```python
from build123d import *

# Parameters (mm, degrees)
BASPROSKE_W             = 10
BASPROSKE_H             = 19
TOOTHCUT_DEPTH          = 29.670542374
TEETHCUTS_COUNT         = 17
TEETHCUTS_ANGLE         = 338.823529412
BORSKE_R                = 2.5
BORE_DEPTH              = 50.0019304
SKETCH1_W               = 10
SKETCH1_H               = 40
CUT_EXTRUDE1_DEPTH      = 20
CUT_EXTRUDE1_DEPTH_BACK = 20
BOSS_EXTRUDE1_DEPTH     = 5
SKETCH5_R               = 1.5
CUT_EXTRUDE5_DEPTH      = 68.251600881
FILLET2_R               = 4.5
SKETCH7_R               = 6
CUT_EXTRUDE7_DEPTH      = 3
CUT_EXTRUDE8_DEPTH      = 2
SKETCH8_R               = 1.5
CUT_EXTRUDE9_DEPTH      = 64.982759166
FILLET3_R               = 4.5


with BuildPart() as part:
    # BasProSke → Base-Revolve (revolve)
    with BuildSketch(Plane(origin=(0, 0, 0), x_dir=(1, 0, 0), z_dir=(0, 1, 0)), mode=Mode.PRIVATE) as base_revolve_sk:
        with Locations((5, 9.5)):
            Rectangle(BASPROSKE_W, BASPROSKE_H)
    revolve(base_revolve_sk.sketch.rotate(Axis((-10, 0, 0), (1, 0, 0)), 180), axis=Axis((-10, 0, 0), (1, 0, 0)))

    # TooCutSke → ToothCut (cut, through all)
    with BuildSketch(Plane(origin=(0, 0, 0), x_dir=(0, 0, -1), z_dir=(1, 0, 0))):
        with BuildLine():
            ThreePointArc((1.020352389, 14.463052306), (0, 14.499), (-1.020352389, 14.463052306))
            ThreePointArc((-1.020352389, 14.463052306), (-1.632621885, 16.804485203), (-3.026143023, 18.783192049))
            ThreePointArc((-3.026143023, 18.783192049), (0, 19.0254), (3.026143023, 18.783192049))
            ThreePointArc((3.026143023, 18.783192049), (1.632621885, 16.804485203), (1.020352389, 14.463052306))
        make_face()
    toothcut = extrude(amount=TOOTHCUT_DEPTH, mode=Mode.SUBTRACT)

    # TeethCuts: ToothCut ×17 about axis
    teethcuts_axis = Axis((-10, 0, 0), (1, 0, 0))
    for i in range(1, TEETHCUTS_COUNT):
        add(toothcut.rotate(teethcuts_axis, i * TEETHCUTS_ANGLE / (TEETHCUTS_COUNT - 1)), mode=Mode.SUBTRACT)

    # BorSke → Bore (cut, symmetric)
    with BuildSketch(Plane(origin=(0, 0, 0), x_dir=(0, 0, -1), z_dir=(1, 0, 0))):
        with Locations(Location((0, 0, 0), (0, 0, 180))):
            Circle(BORSKE_R)
    extrude(amount=BORE_DEPTH, both=True, mode=Mode.SUBTRACT)

    # Sketch1 → Cut-Extrude1 (cut, two sides)
    with BuildSketch(Plane.XY) as cut_extrude1_sk:
        Rectangle(SKETCH1_W, SKETCH1_H)
    extrude(amount=CUT_EXTRUDE1_DEPTH, mode=Mode.SUBTRACT)
    extrude(cut_extrude1_sk.sketch, amount=-CUT_EXTRUDE1_DEPTH_BACK, mode=Mode.SUBTRACT)

    # Sketch4 → Boss-Extrude1 (add)
    with BuildSketch(Plane(origin=(10, 0, 0), x_dir=(0, 0, -1), z_dir=(1, 0, 0))):
        with BuildLine():
            Line((5, 0), (5, 47.113248654))
            Line((5, 47.113248654), (14.820508076, 52.783121635))
            Line((14.820508076, 52.783121635), (14.820508076, 64.330127019))
            Line((14.820508076, 64.330127019), (-5, 52.886751346))
            Line((-5, 52.886751346), (-5, 0))
            Line((-5, 0), (-2.5, 0))
            ThreePointArc((-2.5, 0), (0, 2.5), (2.5, 0))
            Line((2.5, 0), (5, 0))
        make_face()
    extrude(amount=-BOSS_EXTRUDE1_DEPTH)

    # Sketch5 → Cut-Extrude5 (cut, through all)
    with BuildSketch(Plane.ZY.offset(-5)):
        with Locations(Location((-11.320508076, 57.330127019, 0), (0, 0, 270))):
            Circle(SKETCH5_R)
    extrude(amount=-CUT_EXTRUDE5_DEPTH, mode=Mode.SUBTRACT)

    # Fillet2
    fillet2_edges = [part.edges().sort_by_distance(p)[0] for p in [
        (7.5, 64.330127019, -14.820508076),
        (7.5, 52.783121635, -14.820508076),
    ]]
    fillet(fillet2_edges, radius=FILLET2_R)

    # Sketch7 → Cut-Extrude7 (cut)
    with BuildSketch(Plane(origin=(10, 0, 0), x_dir=(0, 0, -1), z_dir=(1, 0, 0))):
        with Locations((11.320508076, 57.330127019)):
            Circle(SKETCH7_R)
    extrude(amount=-CUT_EXTRUDE7_DEPTH, mode=Mode.SUBTRACT)

    # Sketch2 → Cut-Extrude8 (cut)
    with BuildSketch(Plane.ZY.offset(-5)):
        with BuildLine():
            Line((0, -12.5), (0, -4))
            ThreePointArc((0, -4), (-2.624080254, -3.018973803), (-3.961014771, -0.557101411))
            Line((-3.961014771, -0.557101411), (-2, -14.5))
            ThreePointArc((-2, -14.5), (-1.414213562, -13.085786438), (0, -12.5))
        make_face()
        with BuildLine():
            ThreePointArc((2, -14.5), (1.414213562, -13.085786438), (0, -12.5))
            Line((0, -12.5), (0, -16.5))
            ThreePointArc((0, -16.5), (1.414213562, -15.914213562), (2, -14.5))
        make_face()
        with BuildLine():
            Line((0, -16.5), (0, -12.5))
            ThreePointArc((0, -12.5), (-1.414213562, -13.085786438), (-2, -14.5))
            ThreePointArc((-2, -14.5), (-1.414213562, -15.914213562), (0, -16.5))
        make_face()
        with BuildLine():
            ThreePointArc((3.850641774, -1.082847141), (2.415430752, -3.188368593), (0, -4))
            Line((0, -4), (0, -12.5))
            ThreePointArc((0, -12.5), (1.414213562, -13.085786438), (2, -14.5))
            Line((2, -14.5), (3.850641774, -1.082847141))
        make_face()
        with BuildLine():
            ThreePointArc((-3.961014771, -0.557101411), (-2.624080254, -3.018973803), (0, -4))
            ThreePointArc((0, -4), (2.415430752, -3.188368593), (3.850641774, -1.082847141))
            Line((3.850641774, -1.082847141), (4, 0))
            ThreePointArc((4, 0), (-0.279231906, 3.99024179), (-3.961014771, -0.557101411))
        make_face()
        with BuildLine():
            ThreePointArc((2.5, 0), (1.767766953, -1.767766953), (0, -2.5))
            ThreePointArc((0, -2.5), (-1.767766953, 1.767766953), (2.5, 0))
        make_face(mode=Mode.SUBTRACT)
    extrude(amount=-CUT_EXTRUDE8_DEPTH, mode=Mode.SUBTRACT)

    # Sketch8 → Cut-Extrude9 (cut, through all)
    with BuildSketch(Plane.ZY.offset(-7)):
        with Locations(Location((0, -8.45, 0), (0, 0, 270))):
            Circle(SKETCH8_R)
        with Locations(Location((0, -12.45, 0), (0, 0, 270))):
            Circle(SKETCH8_R)
    extrude(amount=-CUT_EXTRUDE9_DEPTH, mode=Mode.SUBTRACT)

    # Fillet3
    fillet3_edges = [part.edges().sort_by_distance(p)[0] for p in [
        (8.5, 51.449252752, -12.5101794),
    ]]
    fillet(fillet3_edges, radius=FILLET3_R)


solid = part.part
```
Geometry check sheet. Reference: the model listing, model coordinates, mm. A direction names the side the tool comes from. Round coordinates to 2 decimals unless told otherwise and drop trailing zeros. Order: outer loops, then holes, each group sorted by start corner. A loop starts at its lowest first (then second) coordinate and runs counter-clockwise, first axis right, second up. Notation, with made-up numbers: (70, -1.5) - (106, -1.5) arc R11 ccw to (106, 7.5) - close; hole circle Ø7 at (25.25, 84). An arc over 180 degrees is marked (long way). Use a Markdown table: item, result. Add a question column.
(1) Sectioned sample at A-A, the plane y = 40. Enter the section's corners in (x, z), and give its area (3 significant figures).
(2) Tool access check on faces 4 (the cylindrical face through (7.46, 10.72, 9.76)), 5 (the cylindrical face through (7.465, -16.178, -4.664)), 6 (the flat face through (7, -6, 0)), 7 (the cylindrical face through (7.465, 1.352, 14.436)), 8 (the cylindrical face through (5.986, 53.16, -14.234)). Record the directions out of +Z, -Z, +X, -X, +Y, -Y that give a thin tool (end or side, any length) a straight path to the whole face; none if there is none.
(3) Release check for a two-part mould opening along Y. For faces 1 (the cylindrical face through (7.465, -15.098, 7.452)), 2 (the cylindrical face through (7.46, 11.3, 12.48)), 3 (the flat face through (8, 34, 5)) record: pulls with the +Y half, pulls with the -Y half, needs draft (parallel to the pull), parting line crosses it, or undercut.
(4) Sectioned sample at B-B, the plane x = 6. Count the separate pieces of the cut face and the enclosed holes in it, and give its area (3 significant figures).
(5) Material ranges on line 1 along Z through (x, y) = (7.95, -12.45); line 2 along Z through (x, y) = (9.3, -8.45); line 3 along Z through (x, y) = (5.6, -11.5), recorded low to high. Write a range as [from, to].
(6) Depth check by flat-ended pin: pin 1 (3 mm diameter, centred on y = 53.5, z = -11, fed in from +X); pin 2 (6.5 mm diameter, centred on y = -2, z = 0, fed in from -X); pin 3 (0.6 mm diameter, centred on x = 6, y = 56, fed in from -Z). Enter the tip coordinate at first touch or a pass-through.
Answers below:
| question | item | result |
|---|---|---|
| 1 | outline | (5, -5) - (10, -5) - (10, 5) - (5, 5) - close |
| 1 | area | 50.0 mm² |
| 2 | face 4 | +X, -X |
| 2 | face 5 | +X, -X, -Y |
| 2 | face 6 | -X |
| 2 | face 7 | +Z, +X, -X |
| 2 | face 8 | -Z, +X, -X |
| 3 | face 1 | undercut |
| 3 | face 2 | pulls with the +Y half |
| 3 | face 3 | needs draft |
| 4 | separate pieces | 2 |
| 4 | enclosed holes | 1 |
| 4 | area | 1,230 mm² |
| 5 | line 1 | [-12.87, -9.06], [-7.43, -1.5], [1.5, 7.43], [9.06, 12.87] |
| 5 | line 2 | [-17.02, -13.2], [-11.78, -1.5], [1.5, 11.78], [13.2, 17.02] |
| 5 | line 3 | [-12.46, -2.42], [2.41, 12.46] |
| 6 | pin 1 | x = 7 |
| 6 | pin 2 | x = 7 |
| 6 | pin 3 | z = -14.82 |
